Check sheet for the modelled part. Datum: model origin and axes. Units: mm. Face numbers are marked on the shaded views. A direction names the side the tool comes from. Round coordinates to 2 decimals unless told otherwise and drop trailing zeros. Loops run counter-clockwise (first coordinate to the right, second up) from the corner with the lowest first, then second, coordinate; pieces in that order, holes last. Notation, with made-up numbers: (23.5, 31.5) -> (43.5, 31.5) arc R20 cw to (43.5, 58.5) -> close; hole circle Ø2 at (-31.5, -24). An arc over 180 degrees is marked (long way). One line per item, written item: value. Start each with the question number.
1. Material ranges on L1, parallel to Z at x = -45, y = 27.15; L2, parallel to X at y = 27.9, z = -35; L3, parallel to X at y = 19.25, z = -32, recorded low to high.
2. Cross-section at A-A on x = -45. Record the cut outline in (y, z).
3. Go/stop test with flat-tipped pins: pin 1 (6.5 mm diameter, centred on x = -46, z = -38, fed in from -Y); pin 2 (2 mm diameter, centred on y = 9, z = -34, fed in from -X); pin 3 (1.8 mm diameter, centred on x = -34.5, z = -1, fed in from +Y). Record where each tip stops, or that it passes through.
4. Cross-section at B-B on y = 19.5. Record the cut outline in (x, z).
5. Set-up check for the marked faces 1 and 2: record each of +Z, -Z, +X, -X, +Y, -Y from which the full face is reachable in a straight line by a thin tool's end or side.
6. Cross-section at D-D on x = 9. Record the cut outline in (y, z), then the cut area to 3 significant figures.
7. Cross-section at C-C on z = 17.5. Record the cut outline in (x, y), then the cut area to 4 significant figures.
8. Release check for a two-part mould opening along X. For the marked faces 3, 4 and 5 record: +X half, -X half, draft (parallel to the pull), parting line (faces both ways), or undercut.
from build123d import *

# Parameters (mm, degrees)
SKETCH1_W                       = 74
SKETCH1_H                       = 53
BOSS_EXTRUDE1_DEPTH             = 4
SKETCH2_W                       = 3.5
SKETCH2_H                       = 53
BOSS_EXTRUDE2_DEPTH             = 25
CUT_EXTRUDE1_REACH              = 85.781
SKETCH3_W                       = 20
SKETCH3_H                       = 15
SKETCH5_W                       = 20
SKETCH5_H                       = 4
BOSS_EXTRUDE4_DEPTH             = 15
MIRROR4_COPY_1_SKETCH_W         = 20
MIRROR4_COPY_1_SKETCH_H         = 4
MIRROR4_COPY_1_DEPTH            = 15
SKETCH6_W                       = 3.5
SKETCH6_H                       = 15
BOSS_EXTRUDE5_DEPTH             = 25
MIRROR6_COPY_1_SKETCH_W         = 3.5
MIRROR6_COPY_1_SKETCH_H         = 15
MIRROR6_COPY_1_DEPTH            = 25
MIRROR6_COPY_2_SKETCH_W         = 3.5
MIRROR6_COPY_2_SKETCH_H         = 15
MIRROR6_COPY_2_DEPTH            = 25
SKETCH7_W                       = 4.5
SKETCH7_H                       = 12.5
BOSS_EXTRUDE6_DEPTH             = 7
MIRROR8_COPY_1_SKETCH_W         = 4.5
MIRROR8_COPY_1_SKETCH_H         = 12.5
MIRROR8_COPY_1_DEPTH            = 7
SKETCH8_W                       = 13
SKETCH8_H                       = 3.5
BOSS_EXTRUDE7_DEPTH             = 16
MIRROR10_COPY_1_SKETCH_W        = 13
MIRROR10_COPY_1_SKETCH_H        = 3.5
MIRROR10_COPY_1_DEPTH           = 16
CUT_EXTRUDE2_REACH              = 105.263
SKETCH9_W                       = 57
SKETCH9_H                       = 15
F_4_0MM_CLEARANCE_DOWEL_HOLE1_D = 4
FILLET1_R                       = 6.5
FILLET2_R                       = 1
FILLET3_R                       = 1


with BuildPart() as part:
    # Sketch1 → Boss-Extrude1 (new body)
    with BuildSketch(Plane(origin=(0, 0, 0), x_dir=(1, 0, 0), z_dir=(0, 1, 0))):
        Rectangle(SKETCH1_W, SKETCH1_H)
    extrude(amount=BOSS_EXTRUDE1_DEPTH)

    # Sketch2 → Boss-Extrude2 (add)
    with BuildSketch(Plane(origin=(0, 4, 0), x_dir=(1, 0, 0), z_dir=(0, 1, 0))):
        with Locations((-35.25, 0)):
            Rectangle(SKETCH2_W, SKETCH2_H)
    boss_extrude2 = extrude(amount=BOSS_EXTRUDE2_DEPTH)

    # Mirror1: Boss-Extrude2 across plane
    add(boss_extrude2.mirror(Plane(origin=(0, 0, 0), x_dir=(0, 0, 1), z_dir=(1, 0, 0))))

    # Sketch3 → Cut-Extrude1 (cut, up to next)
    with BuildSketch(Plane.ZY.offset(37), mode=Mode.PRIVATE) as cut_extrude1_sk1:
        with Locations((0, 21.5)):
            Rectangle(SKETCH3_W, SKETCH3_H)
    cut_extrude1_tool1 = extrude(cut_extrude1_sk1.sketch, amount=-CUT_EXTRUDE1_REACH, mode=Mode.PRIVATE) & part.part
    add(cut_extrude1_tool1.solids().sort_by_distance((-37, 21.5, 0))[0], mode=Mode.SUBTRACT)

    # Sketch5 → Boss-Extrude4 (add)
    with BuildSketch(Plane(origin=(0, 0, -26.5), x_dir=(-1, 0, 0), z_dir=(0, 0, -1))):
        with Locations((27, 2)):
            Rectangle(SKETCH5_W, SKETCH5_H)
    boss_extrude4 = extrude(amount=BOSS_EXTRUDE4_DEPTH)

    # Mirror3: Boss-Extrude4 across plane
    add(boss_extrude4.mirror(Plane.XY))

    # Mirror4: Boss-Extrude4 across plane
    add(boss_extrude4.mirror(Plane(origin=(0, 0, 0), x_dir=(0, 0, 1), z_dir=(1, 0, 0))))

    # Mirror4 copy 1 sketch → Mirror4 copy 1 (add)
    with BuildSketch(Plane.XY.offset(26.5)):
        with Locations((27, 2)):
            Rectangle(MIRROR4_COPY_1_SKETCH_W, MIRROR4_COPY_1_SKETCH_H)
    extrude(amount=MIRROR4_COPY_1_DEPTH)

    # Sketch6 → Boss-Extrude5 (add)
    with BuildSketch(Plane(origin=(0, 4, 0), x_dir=(1, 0, 0), z_dir=(0, 1, 0))):
        with Locations((-35.25, 34)):
            Rectangle(SKETCH6_W, SKETCH6_H)
    boss_extrude5 = extrude(amount=BOSS_EXTRUDE5_DEPTH)

    # Mirror5: Boss-Extrude5 across plane
    add(boss_extrude5.mirror(Plane.XY))

    # Mirror6 copy 1 sketch → Mirror6 copy 1 (add)
    with BuildSketch(Plane(origin=(0, 4, 0), x_dir=(-1, 0, 0), z_dir=(0, 1, 0))):
        with Locations((-35.25, 34)):
            Rectangle(MIRROR6_COPY_1_SKETCH_W, MIRROR6_COPY_1_SKETCH_H)
    extrude(amount=MIRROR6_COPY_1_DEPTH)

    # Mirror6 copy 2 sketch → Mirror6 copy 2 (add)
    with BuildSketch(Plane(origin=(0, 4, 0), x_dir=(-1, 0, 0), z_dir=(0, 1, 0))):
        with Locations((-35.25, -34)):
            Rectangle(MIRROR6_COPY_2_SKETCH_W, MIRROR6_COPY_2_SKETCH_H)
    extrude(amount=MIRROR6_COPY_2_DEPTH)

    # Sketch7 → Boss-Extrude6 (add)
    with BuildSketch(Plane(origin=(0, 4, 0), x_dir=(1, 0, 0), z_dir=(0, 1, 0))):
        with Locations((-22.25, 35.25)):
            Rectangle(SKETCH7_W, SKETCH7_H)
    boss_extrude6 = extrude(amount=BOSS_EXTRUDE6_DEPTH)

    # Mirror7: Boss-Extrude6 across plane
    add(boss_extrude6.mirror(Plane.XY))

    # Mirror8: Boss-Extrude6 across plane
    add(boss_extrude6.mirror(Plane(origin=(0, 0, 0), x_dir=(0, 0, 1), z_dir=(1, 0, 0))))

    # Mirror8 copy 1 sketch → Mirror8 copy 1 (add)
    with BuildSketch(Plane(origin=(0, 4, 0), x_dir=(-1, 0, 0), z_dir=(0, 1, 0))):
        with Locations((-22.25, 35.25)):
            Rectangle(MIRROR8_COPY_1_SKETCH_W, MIRROR8_COPY_1_SKETCH_H)
    extrude(amount=MIRROR8_COPY_1_DEPTH)

    # Sketch8 → Boss-Extrude7 (add)
    with BuildSketch(Plane.ZY.offset(37)):
        with Locations((-35, 27.25)):
            Rectangle(SKETCH8_W, SKETCH8_H)
    boss_extrude7 = extrude(amount=BOSS_EXTRUDE7_DEPTH)

    # Mirror9: Boss-Extrude7 across plane
    add(boss_extrude7.mirror(Plane.XY))

    # Mirror10: Boss-Extrude7 across plane
    add(boss_extrude7.mirror(Plane(origin=(0, 0, 0), x_dir=(0, 0, 1), z_dir=(1, 0, 0))))

    # Mirror10 copy 1 sketch → Mirror10 copy 1 (add)
    with BuildSketch(Plane(origin=(37, 0, 0), x_dir=(0, 0, -1), z_dir=(1, 0, 0))):
        with Locations((-35, 27.25)):
            Rectangle(MIRROR10_COPY_1_SKETCH_W, MIRROR10_COPY_1_SKETCH_H)
    extrude(amount=MIRROR10_COPY_1_DEPTH)

    # Sketch9 → Cut-Extrude2 (cut, up to next)
    with BuildSketch(Plane(origin=(37, 0, 0), x_dir=(0, 0, -1), z_dir=(1, 0, 0)), mode=Mode.PRIVATE) as cut_extrude2_sk1:
        with Locations((0, 21.5)):
            Rectangle(SKETCH9_W, SKETCH9_H)
    cut_extrude2_tool1 = extrude(cut_extrude2_sk1.sketch, amount=-CUT_EXTRUDE2_REACH, mode=Mode.PRIVATE) & part.part
    add(cut_extrude2_tool1.solids().sort_by_distance((37, 21.5, 0))[0], mode=Mode.SUBTRACT)

    # Ø4.0mm Clearance Dowel Hole1 (through all)
    with Locations(Plane(origin=(0, 25.5, 0), x_dir=(-1, 0, 0), z_dir=(0, -1, 0))):
        with Locations((-45, 35), (-45, -35), (45, 35), (45, -35)):
            Hole(F_4_0MM_CLEARANCE_DOWEL_HOLE1_D / 2)

    # Fillet1
    fillet1_edges = [part.edges().sort_by_distance(p)[0] for p in [
        (-53, 27.25, -41.5),
        (-53, 27.25, -28.5),
        (-53, 27.25, 41.5),
        (-53, 27.25, 28.5),
        (53, 27.25, 41.5),
        (53, 27.25, 28.5),
        (53, 27.25, -41.5),
        (53, 27.25, -28.5),
    ]]
    fillet(fillet1_edges, radius=FILLET1_R - 0.0001)  # a hair under: the kernel refuses the full size

    # Fillet2
    fillet2_edges = [part.edges().sort_by_distance(p)[0] for p in [
        (-33.5, 4, 0),
        (-37, 25.5, -35),
        (-37, 25.5, 35),
        (37, 25.5, 35),
        (37, 25.5, -35),
        (35.25, 14, 28.5),
        (35.25, 14, -28.5),
        (33.5, 4, 0),
        (-35.25, 14, -10),
        (-35.25, 14, 10),
        (-17, 2, -26.5),
        (-17, 2, 26.5),
        (17, 2, 26.5),
        (17, 2, -26.5),
    ]]
    fillet(fillet2_edges, radius=FILLET2_R)

    # Fillet3
    fillet3_edges = [part.edges().sort_by_distance(p)[0] for p in [
        (0, 0, -26.5),
        (0, 0, 26.5),
        (16.707106781, 0, -26.792893219),
        (-16.707106781, 0, -26.792893219),
        (-16.707106781, 0, 26.792893219),
        (16.707106781, 0, 26.792893219),
        (-37, 0, 0),
        (37, 0, 0),
        (-17, 0, -34.5),
        (-17, 0, 34.5),
        (17, 0, 34.5),
        (17, 0, -34.5),
    ]]
    fillet(fillet3_edges, radius=FILLET3_R)


solid = part.part
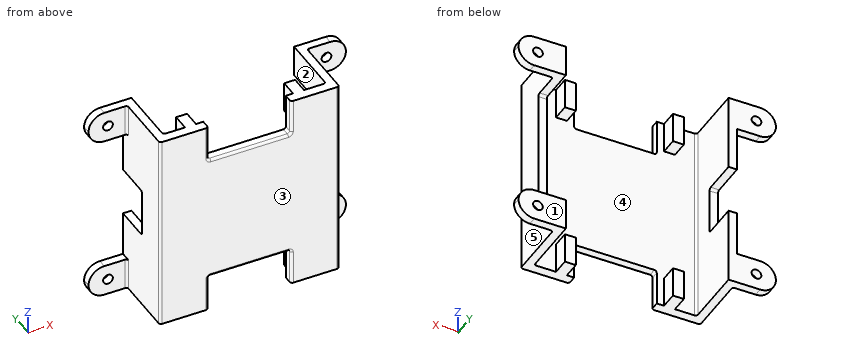
Taken from the geometry:
1. L1: z = -41.5 to -37, -33 to -28.5, 28.5 to 33, 37 to 41.5
1. L2: x = -53 to -47, -43 to -33.5, 33.5 to 43, 47 to 53
1. L3: x = -37 to -33.5, 33.5 to 37
2. outline: (25.5, -41.5) -> (29, -41.5) -> (29, -37) -> (25.5, -37) -> close; (25.5, -33) -> (29, -33) -> (29, -28.5) -> (25.5, -28.5) -> close; (25.5, 28.5) -> (29, 28.5) -> (29, 33) -> (25.5, 33) -> close; (25.5, 37) -> (29, 37) -> (29, 41.5) -> (25.5, 41.5) -> close
3. pin 1: stops at y = 25.5
3. pin 2: stops at x = -37
3. pin 3: stops at y = 14
4. outline: (-37, -41.5) -> (-33.5, -41.5) -> (-33.5, -10) -> (-37, -10) -> close; (-37, 10) -> (-33.5, 10) -> (-33.5, 41.5) -> (-37, 41.5) -> close; (33.5, -41.5) -> (37, -41.5) -> (37, -28.5) -> (33.5, -28.5) -> close; (33.5, 28.5) -> (37, 28.5) -> (37, 41.5) -> (33.5, 41.5) -> close
5. face 1: +Z, -Z, +X, -X, +Y
5. face 2: +Z, -Z, +Y
6. outline: (0, -25.5) arc R1 ccw to (1, -26.5) -> (4, -26.5) -> (4, 26.5) -> (1, 26.5) arc R1 ccw to (0, 25.5) -> close
6. area: 212 mm2
7. outline: (-37, 1) arc R1 ccw to (-36, 0) -> (36, 0) arc R1 ccw to (37, 1) -> (37, 14) -> (33.5, 14) -> (33.5, 5) arc R1 cw to (32.5, 4) -> (-32.5, 4) arc R1 cw to (-33.5, 5) -> (-33.5, 29) -> (-37, 29) -> close
7. area: 418.5 mm2
8. face 3: draft
8. face 4: undercut
8. face 5: +X half
